from build123d import *

# Parameters (mm, degrees)
SKETCH1_W           = 30
SKETCH1_H           = 10.5
BOSS_EXTRUDE1_DEPTH = 3
SKETCH2_W           = 30
SKETCH2_H           = 4
BOSS_EXTRUDE2_DEPTH = 33
FILLET1_R           = 5
SKETCH3_R           = 1.575
CUT_EXTRUDE1_DEPTH  = 37.627346341
SKETCH4_R           = 1.575
CUT_EXTRUDE2_DEPTH  = 37.627346341
SKETCH5_R           = 1.25
CUT_EXTRUDE3_DEPTH  = 41.388736054


with BuildPart() as part:
    # Sketch1 → Boss-Extrude1 (new body)
    with BuildSketch(Plane(origin=(0, 0, 0), x_dir=(0, 0, -1), z_dir=(1, 0, 0))):
        Rectangle(SKETCH1_W, SKETCH1_H)
    extrude(amount=BOSS_EXTRUDE1_DEPTH)

    # Sketch2 → Boss-Extrude2 (add)
    with BuildSketch(Plane(origin=(3, 0, 0), x_dir=(0, 0, -1), z_dir=(1, 0, 0))):
        with Locations((0, -3.25)):
            Rectangle(SKETCH2_W, SKETCH2_H)
    extrude(amount=BOSS_EXTRUDE2_DEPTH)

    # Fillet1
    fillet1_edges = [part.edges().sort_by_distance(p)[0] for p in [
        (36, -3.25, 15),
        (36, -3.25, -15),
    ]]
    fillet(fillet1_edges, radius=FILLET1_R)

    # Sketch3 → Cut-Extrude1 (cut, through all)
    with BuildSketch(Plane(origin=(3, 0, 0), x_dir=(0, 0, -1), z_dir=(1, 0, 0))):
        with Locations((-10.5, 2.05)):
            Circle(SKETCH3_R)
    extrude(amount=-CUT_EXTRUDE1_DEPTH, mode=Mode.SUBTRACT)

    # Sketch4 → Cut-Extrude2 (cut, through all)
    with BuildSketch(Plane(origin=(3, 0, 0), x_dir=(0, 0, -1), z_dir=(1, 0, 0))):
        with Locations((10.5, 2.05)):
            Circle(SKETCH4_R)
    extrude(amount=-CUT_EXTRUDE2_DEPTH, mode=Mode.SUBTRACT)

    # Sketch5 → Cut-Extrude3 (cut, through all)
    with BuildSketch(Plane(origin=(0, -5.25, 0), x_dir=(-1, 0, 0), z_dir=(0, -1, 0))):
        with Locations(Location((-24.5, 0, 0), (0, 0, 90))):
            Circle(SKETCH5_R)
    extrude(amount=-CUT_EXTRUDE3_DEPTH, mode=Mode.SUBTRACT)


solid = part.part
Source: CAD feature listing. Evaluate the final solid. Frame: model axes, mm. Round coordinates to 2 decimals unless told otherwise and drop trailing zeros. Loops run counter-clockwise (first coordinate to the right, second up) from the corner with the lowest first, then second, coordinate; pieces in that order, holes last. Notation, with made-up numbers: (61, 66.25) - (118, 66.25) arc R23 cw to (118, 90.25) - close; hole circle Ø7 at (-39.75, 79). An arc over 180 degrees is marked (long way). Write item = value, one per line. Start each with the question number.
Item 1: Section query C-C on z = -10.5. Output: boundary loops of the cut face in (x, y) (3 decimals).
Item 2: Section query A-A on x = 24.5. Output: boundary loops of the cut face in (y, z), plus the area to 3 significant figures.
Item 3: Material intervals for line 1 (X direction, y = -2.85, z = 0); line 2 (Y direction, x = 1.4, z = -10.5) (3 decimals); line 3 (Y direction, x = 20.5, z = 13.25), sorted ascending.
Item 4: Mould query, pull axis X, two halves, no side actions, for faces 1 (the face through (3, 2, 0)), 2 (the face through (19, -1.25, 0)), 3 (the face through (23.28, -3.28, 0.27)). Classes: released by +X, released by -X, zero draft, split by the parting line, or undercut.
Item 5: Section query B-B on y = 2.5. Output: boundary loops of the cut face in (x, z).
Item 6: Section query D-D on z = -7. Output: boundary loops of the cut face in (x, y), plus the area to 4 significant figures.
Item 7: First-contact query: pin 1 Ø3 at (x, y) = (12.5, 0.5) entering from -Z; pin 2 Ø1 at (y, z) = (1.5, 0) entering from +X; pin 3 Ø6 at (x, y) = (29, -0.5) entering from -Z. Flat tips, straight axial feed; report the tip coordinate or a pass-through.
Results list:
q1.outline = (0, -5.25) - (35.975, -5.25) - (35.975, -1.25) - (3, -1.25) - (3, 0.475) - (0, 0.475) - close; (0, 3.625) - (3, 3.625) - (3, 5.25) - (0, 5.25) - close
q2.outline = (-5.25, -15) - (-1.25, -15) - (-1.25, -1.25) - (-5.25, -1.25) - close; (-5.25, 1.25) - (-1.25, 1.25) - (-1.25, 15) - (-5.25, 15) - close
q2.area = 110 mm²
q3.line_1 = 0 to 23.25, 25.75 to 36
q3.line_2 = -5.25 to 0.475, 3.625 to 5.25
q3.line_3 = -5.25 to -1.25
q4.face_1 = released by +X
q4.face_2 = zero draft
q4.face_3 = undercut
q5.outline = (0, -15) - (3, -15) - (3, -12.01) - (0, -12.01) - close; (0, -8.99) - (3, -8.99) - (3, 8.99) - (0, 8.99) - close; (0, 12.01) - (3, 12.01) - (3, 15) - (0, 15) - close
q6.outline = (0, -5.25) - (36, -5.25) - (36, -1.25) - (3, -1.25) - (3, 5.25) - (0, 5.25) - close
q6.area = 163.5 mm²
q7.pin_1 = through
q7.pin_2 = 3
q7.pin_3 = -15
